Could you check a few things on this drawing? It's one solid part, dimensions in mm from its lowest x, y, z. A direction names the side the tool comes from. Round coordinates to 2 decimals unless told otherwise and drop trailing zeros. Write each loop counter-clockwise with the first axis right and the second up, starting at its lowest first coordinate (ties: lowest second). Pieces come first, ordered by that corner, then holes. Notation, with made-up numbers: (-22, -5.5) -> (-7, -5.5) arc R23 cw to (-7, 16.5) -> close; hole circle Ø2 at (29.25, 41). An arc over 180 degrees is marked (long way). Put each result on its own line as item: value. Start each with the question number.
1) I want a section at C-C, the plane z = 11.08. List the corners of the cut face in (x, y) for me.
2) If I drill on line 1 along X through (y, z) = (2.2, 11.08); line 2 along Z through (x, y) = (9.25, 3.75); line 3 along X through (y, z) = (4.65, 5.5), over which ranges is the centre line in solid material (lowest first)? Write a range as [from, to].
3) I want a section at B-B, the plane x = 16.58. List the corners of the cut face in (y, z) for me, then the cut area to 3 significant figures.
4) We'd pull the mould along X, two halves only. Please class the marked faces 3, 4 and 5: released by +X, released by -X, zero draft, split by the parting line, or undercut.
5) I want a section at A-A, the plane y = 1.05. Give the number of separate pieces and of enclosed holes in the cut face, then the cut area to 3 significant figures.
6) Which directions (+Z, -Z, +X, -X, +Y, -Y) give clear straight access to the entire face, cutting with the end or side of a thin tool? Please do the marked faces 1 and 2.
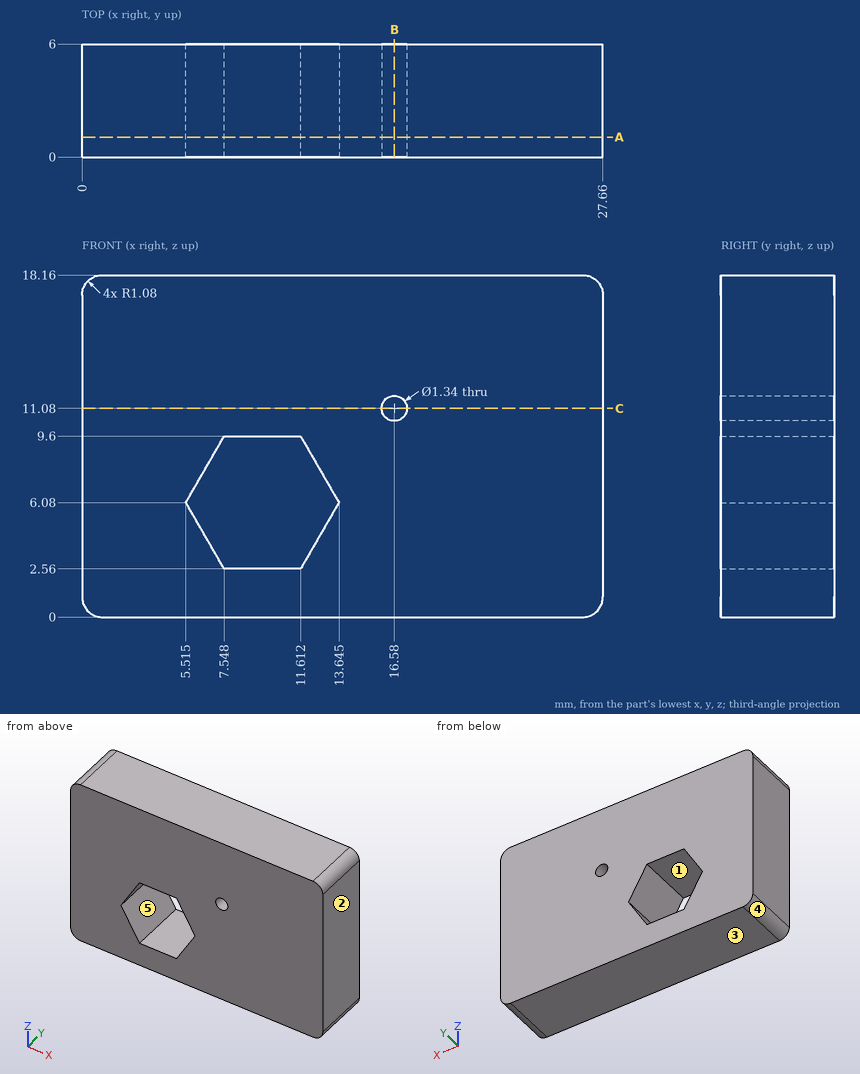
Findings:
1. outline: (0, 0) -> (15.91, 0) -> (15.91, 6) -> (0, 6) -> close; (17.25, 0) -> (27.66, 0) -> (27.66, 6) -> (17.25, 6) -> close
2. line 1: x = [0, 15.91], [17.25, 27.66]
2. line 2: z = [0, 2.56], [9.6, 18.16]
2. line 3: x = [0, 5.85], [13.31, 27.66]
3. outline: (0, 0) -> (6, 0) -> (6, 10.41) -> (0, 10.41) -> close; (0, 11.75) -> (6, 11.75) -> (6, 18.16) -> (0, 18.16) -> close
3. area: 101 mm2
4. face 3: zero draft
4. face 4: released by -X
4. face 5: undercut
5. separate pieces: 1
5. enclosed holes: 2
5. area: 457 mm2
6. face 1: +Y, -Y
6. face 2: +Z, -Z, +X, +Y, -Y
